Model file for the job. Use its own axes, mm. A direction names the side the tool comes from. Round coordinates to 2 decimals unless told otherwise and drop trailing zeros. Order: outer loops, then holes, each group sorted by start corner. A loop starts at its lowest first (then second) coordinate and runs counter-clockwise, first axis right, second up. Notation, with made-up numbers: M 11,63.25 L 16,63.25 A15 cw 16,83.25 Z; hole C 83,60 d5. An arc over 180 degrees is marked long. Return JSON: item names as keys, results as strings. Group by question number.
Item 1: Which spindle directions (+Z, -Z, +X, -X, +Y, -Y) get a long thin tool onto all of the face, cutting with end or side? Do faces 4 (the face through (-5, 15, 2)), 5 (the face through (87, 25.05, 2)), 6 (the face through (-2, 4.95, 2)), 7 (the face through (87, 4.95, 2)), 8 (the face through (-2, 25.05, 2)). Say none if no direction does.
Item 2: Pin check, flat tips, straight feed: pin 1 Ø3 at (x, z) = (44.5, 2) entering from -Y; pin 2 Ø1.5 at (y, z) = (28, 2) entering from +X; pin 3 Ø2 at (x, z) = (-1.5, 3.5) entering from +Y. Stop position of each tip, or through.
Item 3: Probe line 1 along X through (y, z) = (2.5, 2.8). List the from-to ranges inside material, lowest first.
Item 4: Pull direction X, two halves, no side cores. Call faces 1 (the face through (90, 15, 2)), 2 (the face through (0, 28, 2)), 3 (the face through (42, 15, 5)): pulls with the +X half, pulls with the -X half, needs draft (parallel to the pull), parting line crosses it, or undercut.
Item 5: Slice it at A-A on z = 1.7. Write the cut outline in (x, y).
from build123d import *

# Parameters (mm, degrees)
BOSS_EXTRUDE1_DEPTH = 5
FILLET1_R           = 1


with BuildPart() as part:
    # Sketch1 → Boss-Extrude1 (new body)
    with BuildSketch(Plane.XY):
        Polygon((85, 25.05), (85, 30), (0, 30), (0, 25.05), (-5, 25.05), (-5, 4.95), (0, 4.95), (0, 0), (85, 0), (85, 4.95), (90, 4.95), (90, 25.05), align=None)
    extrude(amount=BOSS_EXTRUDE1_DEPTH)

    # Fillet1
    fillet1_edges = [part.edges().sort_by_distance(p)[0] for p in [
        (-5, 4.95, 2.5),
        (-5, 25.05, 2.5),
        (90, 25.05, 2.5),
        (90, 4.95, 2.5),
    ]]
    fillet(fillet1_edges, radius=FILLET1_R)


solid = part.part
Output values:
{
 "1": {"face 4": "+Z, -Z, -X, +Y, -Y", "face 5": "+Z, -Z, +X, +Y", "face 6": "+Z, -Z, -X, -Y", "face 7": "+Z, -Z, +X, -Y", "face 8": "+Z, -Z, -X, +Y"},
 "2": {"pin 1": "y = 0", "pin 2": "x = 85", "pin 3": "y = 25.05"},
 "3": {"line 1": "0 to 85"},
 "4": {"face 1": "pulls with the +X half", "face 2": "pulls with the -X half", "face 3": "needs draft"},
 "5": {"outline": "M -5,5.95 A1 ccw -4,4.95 L 0,4.95 L 0,0 L 85,0 L 85,4.95 L 89,4.95 A1 ccw 90,5.95 L 90,24.05 A1 ccw 89,25.05 L 85,25.05 L 85,30 L 0,30 L 0,25.05 L -4,25.05 A1 ccw -5,24.05 Z"}
}
